The listing builds one solid part. Answer for the finished solid, in the listing's coordinates (mm). Face numbers are marked on the shaded views. A direction names the side the tool comes from. Give positions to 0.01 mm unless a question says otherwise; leave off trailing zeros. Write each loop counter-clockwise with the first axis right and the second up, starting at its lowest first coordinate (ties: lowest second). Pieces come first, ordered by that corner, then holes. Notation, with made-up numbers: (78.5, 4) - (122.5, 4) arc R29 cw to (122.5, 27) - close; hole circle Ø9 at (52.25, -3). An arc over 180 degrees is marked (long way). One line per item, written item: value. Start each with the question number.
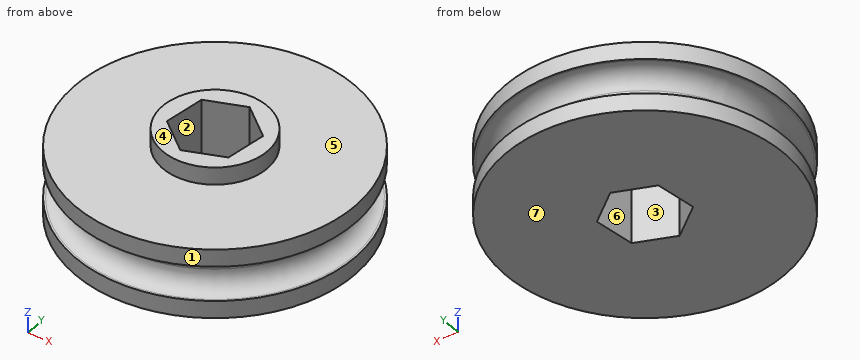
from build123d import *

# Parameters (mm, degrees)
SKETCH1_R           = 25.4
BOSS_EXTRUDE1_DEPTH = 12.7
CUT_EXTRUDE1_START  = -6.35
SKETCH2_R           = 25.4
SKETCH2_R_2         = 21.844
CUT_EXTRUDE1_DEPTH  = 6.35
FILLET1_R           = 3.175
CUT_EXTRUDE4_DEPTH  = 12.7
SKETCH6_R           = 9.525
BOSS_EXTRUDE4_DEPTH = 3.175


with BuildPart() as part:
    # Sketch1 → Boss-Extrude1 (new body)
    with BuildSketch(Plane.XY):
        Circle(SKETCH1_R)
    extrude(amount=BOSS_EXTRUDE1_DEPTH)

    # Sketch2 → Cut-Extrude1 (cut)
    with BuildSketch(Plane.XY.offset(9.525).offset(CUT_EXTRUDE1_START)):
        Circle(SKETCH2_R)
        Circle(SKETCH2_R_2, mode=Mode.SUBTRACT)
    extrude(amount=CUT_EXTRUDE1_DEPTH, mode=Mode.SUBTRACT)

    # Fillet1
    fillet1_edges = [part.edges().sort_by_distance(p)[0] for p in [
        (-21.844, 0, 3.175),
        (-21.844, 0, 9.525),
    ]]
    fillet(fillet1_edges, radius=FILLET1_R - 0.0001)  # a hair under: the kernel refuses the full size

    # Sketch3 → Cut-Extrude4 (cut)
    with BuildSketch(Plane.XY.offset(12.7)):
        Polygon((-1.272676276, -7.221054523), (5.617278521, -4.712697248), (6.889954797, 2.508357276), (1.272676276, 7.221054523), (-5.617278521, 4.712697248), (-6.889954797, -2.508357276), align=None)
    extrude(amount=-CUT_EXTRUDE4_DEPTH, mode=Mode.SUBTRACT)

    # Sketch6 → Boss-Extrude4 (add)
    with BuildSketch(Plane.XY.offset(12.7)):
        Circle(SKETCH6_R)
        Polygon((-1.272676276, -7.221054523), (5.617278521, -4.712697248), (6.889954797, 2.508357276), (1.272676276, 7.221054523), (-5.617278521, 4.712697248), (-6.889954797, -2.508357276), align=None, mode=Mode.SUBTRACT)
    extrude(amount=BOSS_EXTRUDE4_DEPTH)


solid = part.part
Item 1: Straight lines are drawn through the part: line 1 along Y through (x, z) = (-5.5, 1); line 2 along Z through (x, y) = (-15, 7.5); line 3 along Y through (x, z) = (-1, 2.75). For each, find the intervals that lie inside material, in ascending order.
Item 2: For the marked faces 5, 6 and 7, determine the directions among +Z, -Z, +X, -X, +Y, -Y from which every point of the face is accessible in a straight line to the end or side of a thin tool.
Item 3: The mould has two halves that part along X. Classify the marked faces 1, 2, 3 and 4: +X half, -X half, draft (parallel to the pull), parting line (faces both ways), or undercut.
Item 4: Each of these flat-tipped pins is pushed along its axis until it touches: pin 1 Ø4 at (x, z) = (-15, 13) entering from -Y; pin 2 Ø1 at (y, z) = (16, 13.5) entering from +X; pin 3 Ø5 at (y, z) = (-18, 3.5) entering from +X; pin 4 Ø4 at (x, y) = (11.5, -10) entering from +Z. Where does it stop, or does it pass through?
Item 5: Find section A-A on z = 10.5. Determine the outline of the cut face in (x, y), plus the area to 3 significant figures.
Values:
1. line 1: -24.8 to -3.67, 4.76 to 24.8
1. line 2: 0 to 12.7
1. line 3: -25.38 to -7.12, 6.39 to 25.38
2. face 5: +Z
2. face 6: +Z, -Z
2. face 7: -Z, +X, -X, +Y, -Y
3. face 1: parting line
3. face 2: undercut
3. face 3: undercut
3. face 4: draft
4. pin 1: y = -21.81
4. pin 2: through
4. pin 3: x = 20.11
4. pin 4: z = 12.7
5. outline: circle Ø50.8 at (0, 0); hole (-6.89, -2.51) - (-1.27, -7.22) - (5.62, -4.71) - (6.89, 2.51) - (1.27, 7.22) - (-5.62, 4.71) - close
5. area: 1,890 mm^2
